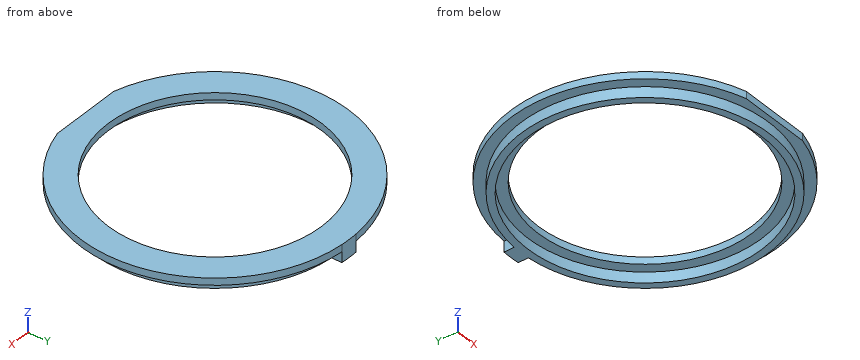
Autodesk Inventor part; units mm, degrees
ref_plane "РабПлоскость1" through (0, 0, -3) normal (0, 0, 1) x (1, 0, 0)
ref_plane "РабПлоскость2" through (-38, -36.68, 0) normal (0, 0, 1) x (1, 0, 0)
ref_plane "YZ Plane" through (0, 0, 0) normal (1, 0, 0) x (0, 1, 0)
ref_plane "РабПлоскость1" through (0, 0, -3) normal (0, 0, 1) x (1, 0, 0)
sketch "Эскиз1" plane through (0, 0, -3) normal (0, 0, 1) x (1, 0, 0)
  circle A0 centre (0, 0) radius 33.125
  arc A1 (-2.5, 35.0359) -> (2.5, 35.0359) centre (0, 0) ccw
  line L0 (2.5, 37.9177) -> (2.5, 35.0359)
  line L1 (-2.5, 35.0359) -> (-2.5, 37.9177)
  arc A2 (2.5, 37.9177) -> (-2.5, 37.9177) centre (0, 0) ccw
  point P0 (2.5, 35.0359)
ref_plane "РабПлоскость2" through (-38, -36.68, 0) normal (0, 0, 1) x (1, 0, 0)
extrude "Выдавливание1" add sketch "Эскиз1" along normal up to surface (3 mm away)
sketch "Эскиз2" plane through (0, 0, 0) normal (0, 0, 1) x (1, 0, 0)
  circle A0 centre (0, 0) radius 30.25
  arc A1 (-2.5, 37.9177) -> (-9.9286, -36.68) centre (0, 0) ccw
  arc A2 (9.9286, -36.68) -> (2.5, 37.9177) centre (0, 0) ccw
  arc A3 (2.5, 37.9177) -> (-2.5, 37.9177) centre (0, 0) ccw
  line L0 (9.9286, -36.68) -> (-9.9286, -36.68)
  point P0 (-2.5, 37.9177)
extrude "Выдавливание2" add sketch "Эскиз2" along normal blind 2
properties part number "ring"
For this review, take the finished solid that the model builds, in its own axes (mm). Coordinates: 2 decimals unless noted, no trailing zeros. Write each loop counter-clockwise with the first axis right and the second up, starting at its lowest first coordinate (ties: lowest second). Pieces come first, ordered by that corner, then holes. Notation, with made-up numbers: (21, 85) - (69, 85) arc R10 cw to (69, 100) - close; hole circle Ø8 at (4.25, -24). An arc over 180 degrees is marked (long way). Answer in a Markdown table with one row per item. Add a question column.
Q1. We need section D-D, the plane y = -16. State the section outline as (x, z) points.
Q2. We need section A-A, the plane x = 0. State the section outline as (y, z) points (3 decimals), and give its area (3 significant figures).
Q3. We need section B-B, the plane y = 0. State the section outline as (x, z) points (3 decimals).
Q4. For P1, Ø22.5, axis at x = -11.5, y = -8.5, coming from the -Z side; P2, Ø1.4, axis at y = 36.5, z = -2, coming from the +X side; P3, Ø1, axis at y = 29, z = -2, coming from the +X side; P4, Ø2, axis at y = -17.5, z = -2, coming from the -X side, all flat-tipped, find the tip position at first contact; note any pin that passes through.
Q5. For probe 1 along Y at (x, z) = (0, -1.05) (3 decimals); probe 2 along Y at (x, z) = (12.5, -1.1); probe 3 along X at (y, z) = (12, 0.75), list the stretches that pass through material, from the lowest coordinate up.
Q6. We need section C-C, the plane z = -2.1. State the section outline as (x, y) points (3 decimals).
Answer list:
| question | item | result |
|---|---|---|
| 1 | outline | (-34.47, 0) - (-31.27, 0) - (-31.27, -3) - (-29, -3) - (-29, 0) - (-25.67, 0) - (-25.67, 2) - (-34.47, 2) - close; (25.67, 0) - (29, 0) - (29, -3) - (31.27, -3) - (31.27, 0) - (34.47, 0) - (34.47, 2) - (25.67, 2) - close |
| 2 | outline | (-36.68, 0) - (-35.125, 0) - (-35.125, -3) - (-33.125, -3) - (-33.125, 0) - (-30.25, 0) - (-30.25, 2) - (-36.68, 2) - close; (30.25, 0) - (33.125, 0) - (33.125, -3) - (38, -3) - (38, 2) - (30.25, 2) - close |
| 2 | area | 49.0 mm2 |
| 3 | outline | (-38, 0) - (-35.125, 0) - (-35.125, -3) - (-33.125, -3) - (-33.125, 0) - (-30.25, 0) - (-30.25, 2) - (-38, 2) - close; (30.25, 0) - (33.125, 0) - (33.125, -3) - (35.125, -3) - (35.125, 0) - (38, 0) - (38, 2) - (30.25, 2) - close |
| 4 | P1 | passes through |
| 4 | P2 | stops at x = 2.5 |
| 4 | P3 | stops at x = 20.53 |
| 4 | P4 | stops at x = -31.01 |
| 5 | probe 1 | y = -35.125 to -33.125, 33.125 to 38 |
| 5 | probe 2 | y = -32.83 to -30.68, 30.68 to 32.83 |
| 5 | probe 3 | x = -36.06 to -27.77, 27.77 to 36.06 |
| 6 | outline | (-2.5, 35.036) arc R35.125 ccw (long way) to (2.5, 35.036) - (2.5, 37.918) arc R38 ccw to (-2.5, 37.918) - close; hole circle Ø66.25 at (0, 0) |
